Read the model definition and answer for the solid it produces. Units are mm, in the model's axes. A direction names the side the tool comes from. Give positions to 0.01 mm unless a question says otherwise; leave off trailing zeros. Order: outer loops, then holes, each group sorted by start corner. A loop starts at its lowest first (then second) coordinate and runs counter-clockwise, first axis right, second up. Notation, with made-up numbers: (-18, 19) -> (24, 19) arc R9 ccw to (24, 33) -> close; hole circle Ø1 at (69, 56.25). An arc over 180 degrees is marked (long way). Answer as CSV lines item,"result". Start each with the question number.
1) Straight lines are drawn through the part: L1, parallel to X at y = 29.5, z = 21.75; L2, parallel to Y at x = 14.5, z = 22.25; L3, parallel to X at y = 50, z = 21.5. For each, find the intervals that lie inside material, in ascending order. Write a range as from..to.
2) Find section D-D (z = 19.5). Determine the outline of the cut face in (x, y).
3) Find section B-B (x = -22.5). Determine the outline of the cut face in (y, z), and give its area (3 significant figures).
4) For faces 1 (the face through (21, -13.141, 20)), 2 (the face through (2, 33, 21.7)), 3 (the face through (-30.24, 53.16, 20.1)), determine the directions among +Z, -Z, +X, -X, +Y, -Y from which every point of the face is accessible in a straight line to the end or side of a thin tool.
5) Find section C-C (y = 11.5). Determine the outline of the cut face in (x, z), and give its area (3 significant figures).
6) Flat-ended cylindrical pins translate along their axes: pin 1 Ø15.5 at (x, y) = (-10.5, 29) entering from -Z; pin 2 Ø0.8 at (x, y) = (9, 47) entering from -Z. Find the tip coordinate at first contact, or state that the pin passes through.
7) Find section A-A (y = 30.5). Determine the outline of the cut face in (x, z).
Autodesk Inventor part; units mm, degrees
ref_plane "YZ Plane" through (0, 0, 0) normal (1, 0, 0) x (0, 1, 0)
ref_plane "XZ Plane" through (0, 0, 0) normal (0, 1, 0) x (-1, 0, 0)
ref_plane "XY Plane" through (0, 0, 0) normal (0, 0, 1) x (1, 0, 0)
sketch "Sketch1" plane through (0, 0, 0) normal (0, 0, 1) x (1, 0, 0)
  line L0 (-34.1779, 55.6594) -> (21.8221, 55.6594)
  line L1 (21.8221, 55.6594) -> (21.8221, -30.6406)
  line L2 (21.8221, -30.6406) -> (-34.1779, -30.6406)
  line L3 (-34.1779, -30.6406) -> (-34.1779, 55.6594)
  point P0 (0, 0)
  dimension "d0" = 56
  dimension "d1" = 86.3
extrude "Extrusion1" add sketch "Sketch1" along normal blind 2
sketch "Sketch2" plane through (0, 0, 2) normal (0, 0, 1) x (1, 0, 0)
  line L0 (-34.1779, 55.6594) -> (21.8221, 55.6594)
  line L1 (21.8221, 55.6594) -> (21.8221, -30.6406)
  line L2 (21.8221, -30.6406) -> (-34.1779, -30.6406)
  line L3 (-34.1779, -30.6406) -> (-34.1779, 55.6594)
  line L4 (-32.1779, 53.6594) -> (19.8221, 53.6594)
  line L5 (19.8221, 53.6594) -> (19.8221, -28.6406)
  line L6 (19.8221, -28.6406) -> (-32.1779, -28.6406)
  line L7 (-32.1779, -28.6406) -> (-32.1779, 53.6594)
  point P0 (0, 0)
  dimension "d4" = 2
  dimension "d5" = 2
  dimension "d6" = 2
  dimension "d7" = 2
extrude "Extrusion2" add sketch "Sketch2" along normal blind 14.4
sketch "Sketch3" plane through (0, 0, 2) normal (0, 0, 1) x (1, 0, 0)
  line L0 (-34.1779, 55.6594) -> (-26.1779, 55.6594)
  line L1 (-26.1779, 55.6594) -> (-26.1779, 47.6594)
  line L2 (-26.1779, 47.6594) -> (-34.1779, 47.6594)
  line L3 (-34.1779, 47.6594) -> (-34.1779, 55.6594)
  line L4 (21.8221, 55.6594) -> (13.8221, 55.6594)
  line L5 (13.8221, 55.6594) -> (13.8221, 47.6594)
  line L6 (13.8221, 47.6594) -> (21.8221, 47.6594)
  line L7 (21.8221, 47.6594) -> (21.8221, 55.6594)
  line L8 (-34.1779, -30.6406) -> (-26.1779, -30.6406)
  line L9 (-26.1779, -30.6406) -> (-26.1779, -22.6406)
  line L10 (-26.1779, -22.6406) -> (-34.1779, -22.6406)
  line L11 (-34.1779, -22.6406) -> (-34.1779, -30.6406)
  line L12 (21.8221, -30.6406) -> (13.8221, -30.6406)
  line L13 (13.8221, -30.6406) -> (13.8221, -22.6406)
  line L14 (13.8221, -22.6406) -> (21.8221, -22.6406)
  line L15 (21.8221, -22.6406) -> (21.8221, -30.6406)
  line L16 (-34.1779, -30.6406) -> (21.8221, -30.6406)
  point P0 (0, 0)
  dimension "d10" = 8
  dimension "d11" = 8
  dimension "d12" = 8
  dimension "d13" = 8
  dimension "d14" = 8
  dimension "d15" = 8
  dimension "d16" = 8
  dimension "d17" = 8
extrude "Extrusion3" add sketch "Sketch3" along normal blind 14.4
sketch "Sketch4" plane through (0, 0, 16.4) normal (0, 0, 1) x (1, 0, 0)
  line L0 (-26.1779, -22.6406) -> (-32.1779, -22.6406)
  line L1 (19.8221, -22.6406) -> (13.8221, -22.6406)
  line L2 (21.8221, 55.6594) -> (21.8221, -30.6406)
  line L3 (21.8221, 55.6594) -> (-34.1779, 55.6594)
  line L4 (-34.1779, -30.6406) -> (-34.1779, 55.6594)
  point P0 (0, 0)
  point P1 (-30.1779, 51.6594)
  point P2 (17.8221, 51.6594)
  point P3 (-30.5754, -26.6406)
  point P4 (17.8221, -26.6406)
  dimension "d20" = 4
  dimension "d21" = 4
  dimension "d22" = 4
  dimension "d23" = 4
  dimension "d24" = 4
  dimension "d25" = 4
  dimension "d26" = 4
hole "Hole1" at (-30.1779, 51.6594, 16.4) at (17.8221, 51.6594, 16.4) at (-30.5754, -26.6406, 16.4) at (17.8221, -26.6406, 16.4) direction (0, 0, -1) diameter 3 depth 6 tip angle 118
fillet "Fillet1" radius 3 4 edges at (-34.1779, 55.6594, 8.2) (21.8221, 55.6594, 8.2) (-34.1779, -30.6406, 8.2) (21.8221, -30.6406, 8.2)
sketch "Sketch5" plane through (0, 0, 2) normal (0, 0, 1) x (1, 0, 0)
  line L0 (-32.1779, 47.6594) -> (19.8221, 47.6594)
  line L1 (19.8221, 47.6594) -> (19.8221, 43.3594)
  line L2 (19.8221, 43.3594) -> (-32.1779, 43.3594)
  line L3 (-32.1779, 43.3594) -> (-32.1779, 47.6594)
  line L4 (19.8221, 47.6594) -> (19.8221, -22.6406)
  line L5 (-32.1779, -22.6406) -> (19.8221, -22.6406)
  line L6 (19.8221, -22.6406) -> (19.8221, -18.3406)
  line L7 (19.8221, -18.3406) -> (-32.1779, -18.3406)
  line L8 (-32.1779, -18.3406) -> (-32.1779, -22.6406)
  point P0 (0, 0)
  dimension "d35" = 4.3
  dimension "d36" = 4.3
extrude "Extrusion4" add sketch "Sketch5" along normal blind 2.5
sketch "Sketch6" plane through (0, 0, 16.4) normal (0, 0, 1) x (1, 0, 0)
  line L0 (-34.1779, 55.6594) -> (21.8221, 55.6594)
  line L1 (21.8221, 55.6594) -> (21.8221, -30.6406)
  line L2 (21.8221, -30.6406) -> (-34.1779, -30.6406)
  line L3 (-34.1779, -30.6406) -> (-34.1779, 55.6594)
  line L4 (18.8221, 55.6594) -> (-31.1779, 55.6594)
  line L5 (-34.1779, 52.6594) -> (-34.1779, -27.6406)
  line L6 (21.8221, -27.6406) -> (21.8221, 52.6594)
  line L7 (-31.1779, -30.6406) -> (18.8221, -30.6406)
  point P0 (0, 0)
extrude "Extrusion5" add sketch "Sketch6" along normal blind 8.5
sketch "Sketch7" plane through (-31.1779, -30.6406, 0) normal (0, -1, 0) x (1, 0, 0)
  line L0 (-3, 16.4) -> (53, 16.4)
  line L1 (53, 16.4) -> (53, 0)
  line L2 (53, 0) -> (-3, 0)
  line L3 (-3, 0) -> (-3, 16.4)
  point P0 (31.1779, 0)
extrude "Extrusion6" cut sketch "Sketch7" against normal blind 300
fillet "Fillet2" radius 3 4 edges at (-34.1779, -30.6406, 20.65) (21.8221, -30.6406, 20.65) (-34.1779, 55.6594, 20.65) (21.8221, 55.6594, 20.65)
sketch "Sketch8" plane through (0, 0, 16.4) normal (0, 0, -1) x (-1, 0, 0)
  line L0 (26.1779, -28.6406) -> (-13.8221, -28.6406)
  line L1 (-13.8221, -28.6406) -> (-13.8221, 53.6594)
  line L2 (-13.8221, 53.6594) -> (26.1779, 53.6594)
  line L3 (26.1779, 53.6594) -> (26.1779, -28.6406)
  line L4 (-19.8221, -22.6406) -> (32.1779, -22.6406)
  line L5 (32.1779, -22.6406) -> (32.1779, 47.6594)
  line L6 (32.1779, 47.6594) -> (-19.8221, 47.6594)
  line L7 (-19.8221, 47.6594) -> (-19.8221, -22.6406)
  line L8 (31.1779, -30.6406) -> (-18.8221, -30.6406)
  line L9 (-18.8221, 55.6594) -> (31.1779, 55.6594)
  line L10 (34.1779, 52.6594) -> (34.1779, -27.6406)
  line L11 (-21.8221, -27.6406) -> (-21.8221, 52.6594)
  point P0 (0, 0)
  dimension "d44" = 8
  dimension "d45" = 8
  dimension "d46" = 8
  dimension "d47" = 8
  dimension "d48" = 2
  dimension "d49" = 2
  dimension "d50" = 2
  dimension "d51" = 2
extrude "Extrusion7" cut sketch "Sketch8" against normal blind 6.5
sketch "Sketch9" plane through (0, 0, 24.9) normal (0, 0, 1) x (1, 0, 0)
  line L0 (-34.1779, 52.6594) -> (-34.1779, -27.6406)
  line L1 (18.8221, 55.6594) -> (-31.1779, 55.6594)
  line L2 (21.8221, -27.6406) -> (21.8221, 52.6594)
  line L3 (-31.1779, -30.6406) -> (18.8221, -30.6406)
  point P0 (0, 0)
  point P1 (-30.1779, 51.6594)
  point P2 (17.8221, 51.6594)
  point P3 (-30.1779, -26.6406)
  point P4 (17.8221, -26.6406)
  dimension "d54" = 4
  dimension "d55" = 4
  dimension "d56" = 4
  dimension "d57" = 4
  dimension "d58" = 4
  dimension "d59" = 4
  dimension "d60" = 4
  dimension "d61" = 4
hole "Hole2" at (-30.1779, 51.6594, 24.9) at (17.8221, 51.6594, 24.9) at (-30.1779, -26.6406, 24.9) at (17.8221, -26.6406, 24.9) direction (0, 0, -1) diameter 3 depth 8 tip angle 118 countersink diameter 6 countersink angle 90
sketch "Sketch10" plane through (21.8221, -27.6406, 24.9) normal (1, 0, 0) x (0, 0, -1)
  line L0 (8.5, 5) -> (8.5, 75.3)
  line L1 (8.5, 14.5) -> (2, 14.5)
  line L2 (2, 14.5) -> (2, 29.5)
  line L3 (2, 29.5) -> (8.5, 29.5)
  line L4 (8.5, 29.5) -> (8.5, 14.5)
  line L5 (0, -3) -> (8.5, -3)
  point P0 (24.9, 27.6406)
  dimension "d69" = 17.5
  dimension "d70" = 32.5
  dimension "d71" = 6.5
extrude "Extrusion8" cut sketch "Sketch10" against normal blind 6.5
sketch "Sketch11" plane through (0, 0, 22.9) normal (0, 0, -1) x (-1, 0, 0)
  line L0 (32.1779, 47.6594) -> (32.1779, -22.6406)
  line L1 (-19.8221, -22.6406) -> (32.1779, -22.6406)
  line L2 (32.1779, -22.6406) -> (32.1779, 47.6594)
  line L3 (32.1779, 47.6594) -> (-19.8221, 47.6594)
  line L4 (-19.8221, 47.6594) -> (-19.8221, -22.6406)
  line L5 (-19.8221, 47.6594) -> (-13.8221, 47.6594)
  point P0 (0, 0)
extrude "Extrusion9" cut sketch "Sketch11" against normal blind 0.8
sketch "Sketch12" plane through (0, 0, 24.9) normal (0, 0, 1) x (1, 0, 0)
  line L0 (-27.7779, 44.9594) -> (-13.9779, 44.9594)
  line L1 (-13.9779, 44.9594) -> (-13.9779, 21.9594)
  line L2 (-13.9779, 21.9594) -> (-27.7779, 21.9594)
  line L3 (-27.7779, 21.9594) -> (-27.7779, 44.9594)
  line L4 (-12.3779, 44.9594) -> (1.4221, 44.9594)
  line L5 (1.4221, 44.9594) -> (1.4221, 21.9594)
  line L6 (1.4221, 21.9594) -> (-12.3779, 21.9594)
  line L7 (-12.3779, 21.9594) -> (-12.3779, 44.9594)
  line L8 (3.0221, 44.9594) -> (16.6221, 44.9594)
  line L9 (16.6221, 44.9594) -> (16.6221, 21.9594)
  line L10 (16.6221, 21.9594) -> (3.0221, 21.9594)
  line L11 (3.0221, 21.9594) -> (3.0221, 44.9594)
  line L12 (18.8221, 55.6594) -> (-31.1779, 55.6594)
  line L13 (-34.1779, 52.6594) -> (-34.1779, -27.6406)
  point P0 (0, 0)
  dimension "d76" = 10.7
  dimension "d77" = 33.7
  dimension "d78" = 6.4
  dimension "d79" = 20.2
  dimension "d80" = 13.8
  dimension "d81" = 13.8
  dimension "d82" = 21.8
  dimension "d83" = 35.6
  dimension "d84" = 37.2
  dimension "d85" = 50.8
  dimension "d86" = 13.6
  dimension "d87" = 1.6
  dimension "d88" = 1.6
extrude "Extrusion10" cut sketch "Sketch12" against normal blind 3
sketch "Sketch13" plane through (0, 0, 23.7) normal (0, 0, -1) x (-1, 0, 0)
  line L0 (-19.8221, 47.6594) -> (32.1779, 47.6594)
  line L1 (-3.0221, 47.6594) -> (-1.4221, 47.6594)
  line L2 (-1.4221, 47.6594) -> (-1.4221, 17.6594)
  line L3 (-1.4221, 17.6594) -> (-3.0221, 17.6594)
  line L4 (-3.0221, 17.6594) -> (-3.0221, 47.6594)
  line L5 (12.3779, 47.6594) -> (13.9779, 47.6594)
  line L6 (13.9779, 47.6594) -> (13.9779, 17.6594)
  line L7 (13.9779, 17.6594) -> (12.3779, 17.6594)
  line L8 (12.3779, 17.6594) -> (12.3779, 47.6594)
  line L9 (-3.0221, 44.9594) -> (-3.0221, 21.9594)
  line L10 (-1.4221, 21.9594) -> (-1.4221, 44.9594)
  line L11 (12.3779, 44.9594) -> (12.3779, 21.9594)
  line L12 (13.9779, 21.9594) -> (13.9779, 44.9594)
  point P0 (0, 0)
  dimension "d91" = 30
extrude "Extrusion11" add sketch "Sketch13" along normal blind 2
sketch "Sketch14" plane through (0, 0, 23.7) normal (0, 0, -1) x (-1, 0, 0)
  line L0 (-19.8221, 47.6594) -> (-3.0221, 47.6594)
  line L1 (-16.6221, 47.6594) -> (-18.2221, 47.6594)
  line L2 (-18.2221, 47.6594) -> (-18.2221, 17.6594)
  line L3 (-18.2221, 17.6594) -> (-16.6221, 17.6594)
  line L4 (-16.6221, 17.6594) -> (-16.6221, 47.6594)
  line L5 (27.7779, 47.6594) -> (29.3779, 47.6594)
  line L6 (29.3779, 47.6594) -> (29.3779, 17.6594)
  line L7 (29.3779, 17.6594) -> (27.7779, 17.6594)
  line L8 (27.7779, 17.6594) -> (27.7779, 47.6594)
  line L9 (-16.6221, 21.9594) -> (-16.6221, 44.9594)
  line L10 (27.7779, 44.9594) -> (27.7779, 21.9594)
  line L11 (-3.0221, 17.6594) -> (-1.4221, 17.6594)
  line L12 (12.3779, 17.6594) -> (13.9779, 17.6594)
  point P0 (0, 0)
  dimension "d94" = 1.6
  dimension "d95" = 1.6
extrude "Extrusion12" add sketch "Sketch14" along normal blind 2
properties part number "cover"
Findings below:
1,L1,"-34.18..-32.18, -29.38..-27.78, -13.98..-12.38, 1.42..3.02, 16.62..18.22, 19.82..21.82"
1,L2,"-30.64..-22.64, 47.66..55.66"
1,L3,"-34.18..-26.18, 13.82..21.82"
2,outline,"(-34.18, -27.64) arc R3 ccw to (-31.18, -30.64) -> (18.82, -30.64) arc R3 ccw to (21.82, -27.64) -> (21.82, -13.14) -> (19.82, -13.14) -> (19.82, -22.64) -> (13.82, -22.64) -> (13.82, -28.64) -> (-26.18, -28.64) -> (-26.18, -22.64) -> (-32.18, -22.64) -> (-32.18, 47.66) -> (-26.18, 47.66) -> (-26.18, 53.66) -> (13.82, 53.66) -> (13.82, 47.66) -> (19.82, 47.66) -> (19.82, 1.86) -> (21.82, 1.86) -> (21.82, 52.66) arc R3 ccw to (18.82, 55.66) -> (-31.18, 55.66) arc R3 ccw to (-34.18, 52.66) -> close; hole circle Ø3 at (-30.18, -26.64); hole circle Ø3 at (-30.18, 51.66); hole circle Ø3 at (17.82, -26.64); hole circle Ø3 at (17.82, 51.66)"
3,outline,"(-30.64, 16.4) -> (-28.64, 16.4) -> (-28.64, 22.9) -> (-22.64, 22.9) -> (-22.64, 23.7) -> (21.96, 23.7) -> (21.96, 24.9) -> (-30.64, 24.9) -> close; (44.96, 23.7) -> (47.66, 23.7) -> (47.66, 22.9) -> (53.66, 22.9) -> (53.66, 16.4) -> (55.66, 16.4) -> (55.66, 24.9) -> (44.96, 24.9) -> close"
3,area,"115 mm²"
4,face 1,"-Z, +X"
4,face 2,"-Z"
4,face 3,"+Z"
5,outline,"(-34.18, 16.4) -> (-32.18, 16.4) -> (-32.18, 23.7) -> (19.82, 23.7) -> (19.82, 16.4) -> (21.82, 16.4) -> (21.82, 24.9) -> (-34.18, 24.9) -> close"
5,area,"96.4 mm²"
6,pin 1,"z = 21.7"
6,pin 2,"z = 23.7"
7,outline,"(-34.18, 16.4) -> (-32.18, 16.4) -> (-32.18, 23.7) -> (-29.38, 23.7) -> (-29.38, 21.7) -> (-27.78, 21.7) -> (-27.78, 24.9) -> (-34.18, 24.9) -> close; (-13.98, 21.7) -> (-12.38, 21.7) -> (-12.38, 24.9) -> (-13.98, 24.9) -> close; (1.42, 21.7) -> (3.02, 21.7) -> (3.02, 24.9) -> (1.42, 24.9) -> close; (16.62, 21.7) -> (18.22, 21.7) -> (18.22, 23.7) -> (19.82, 23.7) -> (19.82, 16.4) -> (21.82, 16.4) -> (21.82, 24.9) -> (16.62, 24.9) -> close"
